Build history of the part. All positions in model axes, mm. A direction names the side the tool comes from. Round coordinates to 2 decimals unless told otherwise and drop trailing zeros. Loops run counter-clockwise (first coordinate to the right, second up) from the corner with the lowest first, then second, coordinate; pieces in that order, holes last.
from build123d import *

# Parameters (mm, degrees)
F1_DEPTH = 3.175
F3_DEPTH = 63.5
F5_DEPTH = 3.175
F6_R     = 5.08


with BuildPart() as f1:
    # F0 (on Front) → F1 (new body)
    with BuildSketch(Plane.XZ):
        with BuildLine():
            Line((0, -24.5087207538), (0, -189.6087207538))
            ThreePointArc((0, -189.6087207538), (98.7828173318, -148.6915380856), (139.7, -49.9087207538))
            ThreePointArc((139.7, -49.9087207538), (119.1365602995, 23.0472248572), (63.5, 74.5253581796))
            Line((63.5, 74.5253581796), (63.5, 38.9912792462))
            ThreePointArc((63.5, 38.9912792462), (44.9012806053, -5.9100013592), (0, -24.5087207538))
        make_face()
        with BuildLine():
            ThreePointArc((-63.5, 74.5253581795), (-135.8299135445, -82.5633465594), (0, -189.6087207538))
            Line((0, -189.6087207538), (0, -24.5087207538))
            ThreePointArc((0, -24.5087207538), (-44.9012806053, -5.9100013592), (-63.5, 38.9912792462))
            Line((-63.5, 38.9912792462), (-63.5, 74.5253581795))
        make_face()
        with BuildLine():
            Line((-152.4, 127.8912792462), (-152.4, -62.8556646327))
            Line((-152.4, -62.8556646327), (-91.2153361462, -189.6087207538))
            Line((-91.2153361462, -189.6087207538), (0, -189.6087207538))
            ThreePointArc((0, -189.6087207538), (-135.8299135445, -82.5633465594), (-63.5, 74.5253581795))
            Line((-63.5, 74.5253581795), (-63.5, 127.8912792462))
            Line((-63.5, 127.8912792462), (-152.4, 127.8912792462))
        make_face()
        with BuildLine():
            ThreePointArc((139.7, -49.9087207538), (98.7828173318, -148.6915380856), (0, -189.6087207538))
            Line((0, -189.6087207538), (91.2153361462, -189.6087207538))
            Line((91.2153361462, -189.6087207538), (152.4, -62.8556646327))
            Line((152.4, -62.8556646327), (152.4, 127.8912792462))
            Line((152.4, 127.8912792462), (63.5, 127.8912792462))
            Line((63.5, 127.8912792462), (63.5, 74.5253581796))
            ThreePointArc((63.5, 74.5253581796), (119.1365602995, 23.0472248572), (139.7, -49.9087207538))
        make_face()
    extrude(amount=F1_DEPTH)

    # F2 (on face) → F3 (join)
    with BuildSketch(Plane.XZ.offset(3.175)):
        Polygon((-149.225, -62.1294560471), (-149.225, 127.8912792462), (-152.4, 127.8912792462), (-152.4, -62.8556646327), (-91.2153361462, -189.6087207538), (91.2153361462, -189.6087207538), (152.4, -62.8556646327), (152.4, 127.8912792462), (149.225, 127.8912792462), (149.225, -62.1294560471), (89.2223863794, -186.4337207538), (-89.2223863794, -186.4337207538), align=None)
    extrude(amount=F3_DEPTH)

    # F4 (on face) → F5 (join)
    with BuildSketch(Plane.XZ.offset(66.675)):
        Polygon((59.3281398768, -138.8087207538), (36.3391902988, -186.4337207538), (89.2223863794, -186.4337207538), (149.225, -62.1294560471), (149.225, 126.3037792462), (101.6, 102.4912792462), (101.6, -51.2363272641), align=None)
        Polygon((-101.6, 102.4912792462), (-149.225, 126.3037792462), (-149.225, -62.1294560471), (-89.2223863794, -186.4337207538), (-36.3391902988, -186.4337207538), (-59.3281398768, -138.8087207538), (-101.6, -51.2363272641), align=None)
        Polygon((36.3391902988, -186.4337207538), (34.8065936602, -189.6087207538), (91.2153361462, -189.6087207538), (152.4, -62.8556646327), (152.4, 127.8912792462), (149.225, 126.3037792462), (149.225, -62.1294560471), (89.2223863794, -186.4337207538), align=None)
        Polygon((-149.225, 126.3037792462), (-152.4, 127.8912792462), (-152.4, -62.8556646327), (-91.2153361462, -189.6087207538), (-34.8065936602, -189.6087207538), (-36.3391902988, -186.4337207538), (-89.2223863794, -186.4337207538), (-149.225, -62.1294560471), align=None)
        Polygon((149.225, 126.3037792462), (152.4, 127.8912792462), (149.225, 127.8912792462), align=None)
        Polygon((-149.225, 127.8912792462), (-152.4, 127.8912792462), (-149.225, 126.3037792462), align=None)
    extrude(amount=F5_DEPTH)

    # F6
    f6_edges = [f1.edges().sort_by_distance(p)[0] for p in [
        (101.6, -68.2625, 102.491279),
        (-101.6, -68.2625, 102.491279),
    ]]
    fillet(f6_edges, radius=F6_R)


solid = f1.part
(1) Slice it at B-B on y = -47. List the corners of the cut face in (x, z) (3 decimals), plus the area to 3 significant figures.
Responses:
outline: (-152.4, -62.856) - (-91.215, -189.609) - (91.215, -189.609) - (152.4, -62.856) - (152.4, 127.891) - (149.225, 127.891) - (149.225, -62.129) - (89.222, -186.434) - (-89.222, -186.434) - (-149.225, -62.129) - (-149.225, 127.891) - (-152.4, 127.891) - close
area: 2,670 mm2
(2) Slice it at A-A on z = 87.5. List the corners of the cut face in (x, y) (3 decimals).
Responses:
outline: (-152.4, -69.85) - (-101.6, -69.85) - (-101.6, -66.675) - (-149.225, -66.675) - (-149.225, -3.175) - (-63.5, -3.175) - (-63.5, 0) - (-152.4, 0) - close; (63.5, -3.175) - (149.225, -3.175) - (149.225, -66.675) - (101.6, -66.675) - (101.6, -69.85) - (152.4, -69.85) - (152.4, 0) - (63.5, 0) - close
(3) Slice it at D-D on z = -156.5. List the corners of the cut face in (x, y) (3 decimals).
Responses:
outline: (-107.197, -69.85) - (-50.788, -69.85) - (-50.788, -66.675) - (-103.672, -66.675) - (-103.672, -3.175) - (103.672, -3.175) - (103.672, -66.675) - (50.788, -66.675) - (50.788, -69.85) - (107.197, -69.85) - (107.197, 0) - (-107.197, 0) - close
(4) Which spindle directions (+Z, -Z, +X, -X, +Y, -Y) get a long thin tool onto all of the face, cutting with end or side? Do faces 1 (the face through (127.13, -68.24, 115.256)), 2 (the face through (-152.4, -34, 34)), 3 (the face through (117, -66.675, -28)). Say none if no direction does.
Responses:
face 1: +Z, -Y
face 2: +Z, -Z, -X, +Y, -Y
face 3: +Z
(5) Probe line 1 (X direction, y = -40, z = 25) (3 decimals); line 2 (Y direction, x = 110, z = 26.5) (3 decimals); line 3 (Z direction, x = 53.5, y = -52). List the from-to ranges inside material, lowest first.
Responses:
line 1: x = -152.4 to -149.225, 149.225 to 152.4
line 2: y = -69.85 to -66.675, -3.175 to 0
line 3: z = -189.61 to -186.43
(6) Pull direction Y, two halves, no side cores. Call faces 4 (the face through (128, -1, 127.891)), 5 (the face through (-2, 0, -29)), 6 (the face through (-119, -66.675, -28)), 7 (the face through (-121, -69.85, -29)): +Y half, -Y half, draft (parallel to the pull), parting line (faces both ways), or undercut.
Responses:
face 4: draft
face 5: +Y half
face 6: undercut
face 7: -Y half
(7) Pin check, flat tips, straight feed: P1, Ø1, axis at x = -14, z = -188.5, coming from the -Y side (3 decimals); P2, Ø5, axis at x = -47.5, y = -44, coming from the +Z side; P3, Ø8, axis at x = 21, z = -98.5, coming from the -Y side (3 decimals). Stop position of each tip, or through.
Responses:
P1: stops at y = -66.675
P2: stops at z = -186.43
P3: stops at y = -3.175
(8) Slice it at C-C on x = 0. List the corners of the cut face in (y, z) (3 decimals).
Responses:
outline: (-66.675, -189.609) - (0, -189.609) - (0, -24.509) - (-3.175, -24.509) - (-3.175, -186.434) - (-66.675, -186.434) - close
